Verification items for this drawing (mm, ordinates from the low corner). A direction names the side the tool comes from. Coordinates: 2 decimals unless noted, no trailing zeros. Order: outer loops, then holes, each group sorted by start corner. A loop starts at its lowest first (then second) coordinate and runs counter-clockwise, first axis right, second up. Notation, with made-up numbers: M 22,-36.75 L 44,-36.75 A15 cw 44,-29.75 Z; hole C 5,-1.5 d7. An arc over 180 degrees is marked long. One line per item, written item: value. Start each with the question number.
1) Sectioned sample at C-C, the plane x = 53. Enter the section's corners in (y, z).
2) Sectioned sample at B-B, the plane z = 16.5. Enter the section's corners in (x, y).
3) Sectioned sample at A-A, the plane y = 54. Enter the section's corners in (x, z).
4) Go/stop test with flat-tipped pins: P1, Ø4, axis at x = 46.5, y = 17, coming from the +Z side; P2, Ø8, axis at x = 45.5, z = 77, coming from the +Y side; P3, Ø16.5, axis at x = 57.5, z = 30.5, coming from the +Y side. Record where each tip stops, or that it passes through.
5) Sectioned sample at D-D, the plane z = 74. Enter the section's corners in (x, y), then the cut area to 3 significant figures.
6) Access from +Z, -Z, +X, -X, +Y, -Y to the whole of each face (thin tool, end or side, straight path). Record for the marked faces 5, 6 and 7.
7) Thickness scan on L1, parallel to Z at x = 53, y = 5.25; L2, parallel to X at y = 5, z = 107; L3, parallel to Y at x = 42, z = 17. Record the ranges inside material, lowest first. Write a range as from..to.
8) Draft check along Y on the marked faces 1, 2, 3 and 4. Enter one of: pulls with the +Y half, pulls with the -Y half, needs draft (parallel to the pull), parting line crosses it, or undercut.
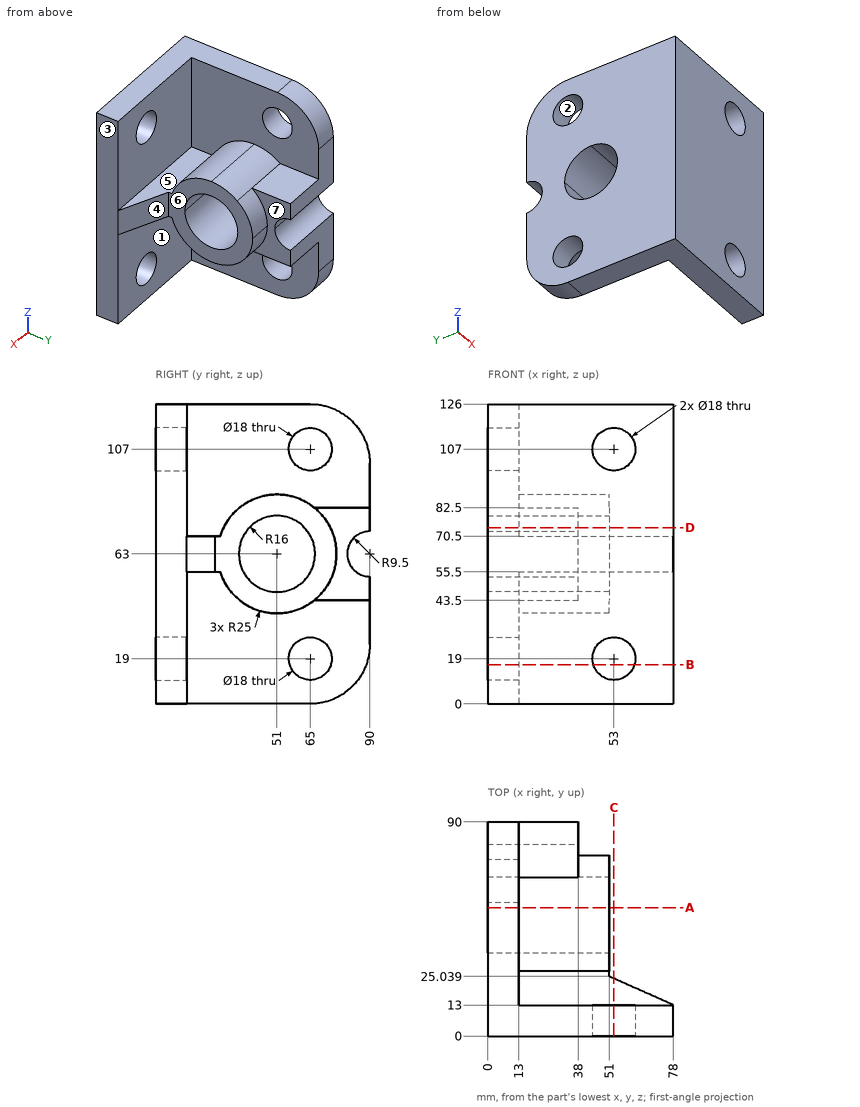
Final values:
1. outline: M 0,0 L 13,0 L 13,10 L 0,10 Z; M 0,28 L 13,28 L 13,55.5 L 24.15,55.5 L 24.15,70.5 L 13,70.5 L 13,98 L 0,98 Z; M 0,116 L 13,116 L 13,126 L 0,126 Z
2. outline: M 0,0 L 44.35,0 L 44.35,13 L 13,13 L 13,56.35 L 0,56.35 Z; M 0,73.65 L 13,73.65 L 13,88.51 L 0,88.51 Z; M 61.65,0 L 78,0 L 78,13 L 61.65,13 Z
3. outline: M 0,0 L 13,0 L 13,38.18 L 51,38.18 L 51,47.28 L 0,47.28 Z; M 0,78.72 L 51,78.72 L 51,87.82 L 13,87.82 L 13,126 L 0,126 Z
4. P1: stops at z = 70.5
4. P2: stops at y = 73.91
4. P3: stops at y = 13
5. outline: M 0,0 L 78,0 L 78,13 L 13,13 L 13,28.55 L 51,28.55 L 51,39.38 L 0,39.38 Z; M 0,62.62 L 51,62.62 L 51,73.45 L 38,73.45 L 38,90 L 0,90 Z
5. area: 2,950 mm^2
6. face 5: +Z, +X
6. face 6: +Z, -Z, +X, +Y
6. face 7: +X, +Y
7. L1: z = 0..10, 28..98, 116..126
7. L2: x = 0..44, 62..78
7. L3: y = 0..13
8. face 1: undercut
8. face 2: undercut
8. face 3: needs draft
8. face 4: pulls with the +Y half
